```python
from build123d import *

# Parameters (mm, degrees)
EXTRUDE_1_DEPTH      = 3
SKETCH_2_R           = 1.5
CUT_EXTRUDE_1_DEPTH  = 3
SKETCH_3_R           = 18.5
SKETCH_3_R_2         = 1.5
CUT_EXTRUDE_2_DEPTH  = 10
SKETCH_4_W           = 90
SKETCH_4_H           = 90
CUT_EXTRUDE_3_DEPTH  = 3
FILLET_3_R           = 6
CHAMFER_1_SIZE       = 8
CUT_EXTRUDE_6_DEPTH  = 10
CHAMFER_2_SIZE       = 15
SKETCH_8_R           = 1.5
CUT_EXTRUDE_7_DEPTH  = 10
SKETCH_9_R           = 1.5
CUT_EXTRUDE_8_DEPTH  = 10
CUT_EXTRUDE_9_DEPTH  = 10
SKETCH_14_R          = 1.5
CUT_EXTRUDE_10_DEPTH = 10
SKETCH_15_R          = 1.5
SKETCH_15_W          = 42
SKETCH_15_H          = 23
CUT_EXTRUDE_11_DEPTH = 10
FILLET_4_R           = 1
SKETCH_16_R          = 1.25
CUT_EXTRUDE_12_DEPTH = 10
SKETCH_19_R          = 1.5
CUT_EXTRUDE_13_DEPTH = 10
SKETCH_20_R          = 1.5
CUT_EXTRUDE_14_DEPTH = 10
SKETCH_21_R          = 1.5
CUT_EXTRUDE_15_DEPTH = 10
SKETCH_22_R          = 1.5
CUT_EXTRUDE_16_DEPTH = 10


with BuildPart() as part:
    # 草图1 → 凸台-拉伸1 (new body)
    with BuildSketch(Plane(origin=(0, 0, 0), x_dir=(1, 0, 0), z_dir=(0, 1, 0))):
        Polygon((-47.5, -71), (-47.5, -125), (47.5, -125), (47.5, -71), (145, -71), (145, 71), (47.5, 71), (47.5, 125), (-47.5, 125), (-47.5, 71), (-145, 71), (-145, -71), align=None)
    extrude(amount=EXTRUDE_1_DEPTH)

    # 草图2 → 切除-拉伸1 (cut)
    with BuildSketch(Plane(origin=(0, 3, 0), x_dir=(1, 0, 0), z_dir=(0, 1, 0))):
        with Locations(Location((110, 62, 0), (0, 0, 270))):
            Circle(SKETCH_2_R)
        with Locations(Location((80, 62, 0), (0, 0, 270))):
            Circle(SKETCH_2_R)
        with Locations(Location((80, 38, 0), (0, 0, 270))):
            Circle(SKETCH_2_R)
        with Locations(Location((110, 38, 0), (0, 0, 270))):
            Circle(SKETCH_2_R)
        with Locations(Location((110, -38, 0), (0, 0, 90))):
            Circle(SKETCH_2_R)
        with Locations(Location((110, -62, 0), (0, 0, 90))):
            Circle(SKETCH_2_R)
        with Locations(Location((80, -38, 0), (0, 0, 90))):
            Circle(SKETCH_2_R)
        with Locations(Location((80, -62, 0), (0, 0, 90))):
            Circle(SKETCH_2_R)
        with Locations(Location((-80, -62, 0), (0, 0, 270))):
            Circle(SKETCH_2_R)
        with Locations(Location((-80, -38, 0), (0, 0, 270))):
            Circle(SKETCH_2_R)
        with Locations(Location((-110, -62, 0), (0, 0, 270))):
            Circle(SKETCH_2_R)
        with Locations(Location((-110, -38, 0), (0, 0, 270))):
            Circle(SKETCH_2_R)
        with Locations(Location((-110, 38, 0), (0, 0, 90))):
            Circle(SKETCH_2_R)
        with Locations(Location((-80, 38, 0), (0, 0, 90))):
            Circle(SKETCH_2_R)
        with Locations(Location((-80, 62, 0), (0, 0, 90))):
            Circle(SKETCH_2_R)
        with Locations(Location((-110, 62, 0), (0, 0, 90))):
            Circle(SKETCH_2_R)
    extrude(amount=-CUT_EXTRUDE_1_DEPTH, mode=Mode.SUBTRACT)

    # 草图3 → 切除-拉伸2 (cut)
    with BuildSketch(Plane(origin=(0, 3, 0), x_dir=(1, 0, 0), z_dir=(0, 1, 0))):
        with Locations(Location((0, 97, 0), (0, 0, 270))):
            Circle(SKETCH_3_R)
        with Locations(Location((29, 117, 0), (0, 0, 270))):
            Circle(SKETCH_3_R_2)
        with Locations(Location((29, 77, 0), (0, 0, 270))):
            Circle(SKETCH_3_R_2)
        with Locations(Location((-29, 77, 0), (0, 0, 270))):
            Circle(SKETCH_3_R_2)
        with Locations(Location((-29, 117, 0), (0, 0, 270))):
            Circle(SKETCH_3_R_2)
    extrude(amount=-CUT_EXTRUDE_2_DEPTH, mode=Mode.SUBTRACT)

    # 草图4 → 切除-拉伸3 (cut)
    with BuildSketch(Plane(origin=(0, 3, 0), x_dir=(1, 0, 0), z_dir=(0, 1, 0))):
        Rectangle(SKETCH_4_W, SKETCH_4_H)
    extrude(amount=-CUT_EXTRUDE_3_DEPTH, mode=Mode.SUBTRACT)

    # 圆角3
    fillet_3_edges = [part.edges().sort_by_distance(p)[0] for p in [
        (-145, 1.5, 71),
        (-145, 1.5, -71),
        (-47.5, 1.5, -125),
        (47.5, 1.5, -125),
        (145, 1.5, -71),
        (145, 1.5, 71),
        (47.5, 1.5, 125),
        (-47.5, 1.5, 125),
    ]]
    fillet(fillet_3_edges, radius=FILLET_3_R)

    # 倒角1
    chamfer_1_edges = [part.edges().sort_by_distance(p)[0] for p in [
        (-47.5, 1.5, 71),
        (-47.5, 1.5, -71),
        (47.5, 1.5, -71),
        (47.5, 1.5, 71),
    ]]
    chamfer(chamfer_1_edges, length=CHAMFER_1_SIZE)

    # 草图7 → 切除-拉伸6 (cut)
    with BuildSketch(Plane(origin=(0, 3, 0), x_dir=(1, 0, 0), z_dir=(0, 1, 0))):
        with BuildLine():
            Line((-65, -20), (-65, 20))
            ThreePointArc((-65, 20), (-58, 27), (-51, 20))
            Line((-51, 20), (-51, -20))
            ThreePointArc((-51, -20), (-58, -27), (-65, -20))
        make_face()
        with BuildLine():
            Line((-141, -15), (-141, 15))
            ThreePointArc((-141, 15), (-137, 19), (-133, 15))
            Line((-133, 15), (-133, -15))
            ThreePointArc((-133, -15), (-137, -19), (-141, -15))
        make_face()
        with BuildLine():
            Line((129, 38), (129, 52))
            ThreePointArc((129, 52), (134, 57), (139, 52))
            Line((139, 52), (139, 38))
            ThreePointArc((139, 38), (134, 33), (129, 38))
        make_face()
        with BuildLine():
            Line((129, -38), (129, -52))
            ThreePointArc((129, -52), (134, -57), (139, -52))
            Line((139, -52), (139, -38))
            ThreePointArc((139, -38), (134, -33), (129, -38))
        make_face()
    extrude(amount=-CUT_EXTRUDE_6_DEPTH, mode=Mode.SUBTRACT)

    # 倒角2
    chamfer_2_edges = [part.edges().sort_by_distance(p)[0] for p in [
        (45, 1.5, -45),
        (45, 1.5, 45),
        (-45, 1.5, 45),
        (-45, 1.5, -45),
    ]]
    chamfer(chamfer_2_edges, length=CHAMFER_2_SIZE)

    # 草图8 → 切除-拉伸7 (cut)
    with BuildSketch(Plane(origin=(0, 3, 0), x_dir=(1, 0, 0), z_dir=(0, 1, 0))):
        with Locations(Location((-139, 50, 0), (0, 0, 270))):
            Circle(SKETCH_8_R)
        with Locations(Location((-131, 50, 0), (0, 0, 270))):
            Circle(SKETCH_8_R)
    extrude(amount=-CUT_EXTRUDE_7_DEPTH, mode=Mode.SUBTRACT)

    # 草图9 → 切除-拉伸8 (cut)
    with BuildSketch(Plane(origin=(0, 3, 0), x_dir=(1, 0, 0), z_dir=(0, 1, 0))):
        with Locations(Location((50.843145751, 56.5, 0), (0, 0, 270))):
            Circle(SKETCH_9_R)
        with Locations(Location((56.5, 50.843145751, 0), (0, 0, 270))):
            Circle(SKETCH_9_R)
        with Locations(Location((56.5, -50.843145751, 0), (0, 0, 270))):
            Circle(SKETCH_9_R)
        with Locations(Location((50.843145751, -56.5, 0), (0, 0, 270))):
            Circle(SKETCH_9_R)
        with Locations(Location((-50.843145751, -56.5, 0), (0, 0, 270))):
            Circle(SKETCH_9_R)
        with Locations(Location((-56.5, -50.843145751, 0), (0, 0, 270))):
            Circle(SKETCH_9_R)
        with Locations(Location((-56.5, 50.843145751, 0), (0, 0, 270))):
            Circle(SKETCH_9_R)
        with Locations(Location((-50.843145751, 56.5, 0), (0, 0, 270))):
            Circle(SKETCH_9_R)
        with Locations(Location((-38, -117, 0), (0, 0, 270))):
            Circle(SKETCH_9_R)
        with Locations(Location((38, -117, 0), (0, 0, 270))):
            Circle(SKETCH_9_R)
    extrude(amount=-CUT_EXTRUDE_8_DEPTH, mode=Mode.SUBTRACT)

    # 草图12 → 切除-拉伸9 (cut)
    with BuildSketch(Plane(origin=(0, 3, 0), x_dir=(1, 0, 0), z_dir=(0, 1, 0))):
        with BuildLine():
            Line((-17.5, -54), (17.5, -54))
            ThreePointArc((17.5, -54), (23.5, -60), (17.5, -66))
            Line((17.5, -66), (-17.5, -66))
            ThreePointArc((-17.5, -66), (-23.5, -60), (-17.5, -54))
        make_face()
    extrude(amount=-CUT_EXTRUDE_9_DEPTH, mode=Mode.SUBTRACT)

    # 草图14 → 切除-拉伸10 (cut)
    with BuildSketch(Plane(origin=(0, 3, 0), x_dir=(1, 0, 0), z_dir=(0, 1, 0))):
        with Locations(Location((36, -69, 0), (0, 0, 270))):
            Circle(SKETCH_14_R)
        with Locations(Location((36, -111, 0), (0, 0, 270))):
            Circle(SKETCH_14_R)
        with Locations(Location((-36, -111, 0), (0, 0, 270))):
            Circle(SKETCH_14_R)
        with Locations(Location((-36, -69, 0), (0, 0, 270))):
            Circle(SKETCH_14_R)
    extrude(amount=-CUT_EXTRUDE_10_DEPTH, mode=Mode.SUBTRACT)

    # 草图15 → 切除-拉伸11 (cut)
    with BuildSketch(Plane(origin=(0, 3, 0), x_dir=(1, 0, 0), z_dir=(0, 1, 0))):
        with Locations(Location((75.36, 5, 0), (0, 0, 270))):
            Circle(SKETCH_15_R)
        with Locations(Location((75.36, -5, 0), (0, 0, 270))):
            Circle(SKETCH_15_R)
        with Locations(Location((124.86, -5, 0), (0, 0, 270))):
            Circle(SKETCH_15_R)
        with Locations(Location((124.86, 5, 0), (0, 0, 270))):
            Circle(SKETCH_15_R)
        with Locations((100.11, 0)):
            Rectangle(SKETCH_15_W, SKETCH_15_H)
    extrude(amount=-CUT_EXTRUDE_11_DEPTH, mode=Mode.SUBTRACT)

    # 圆角4
    fillet_4_edges = [part.edges().sort_by_distance(p)[0] for p in [
        (121.11, 1.5, -11.5),
        (121.11, 1.5, 11.5),
        (79.11, 1.5, 11.5),
        (79.11, 1.5, -11.5),
    ]]
    fillet(fillet_4_edges, radius=FILLET_4_R)

    # 草图16 → 切除-拉伸12 (cut)
    with BuildSketch(Plane(origin=(0, 3, 0), x_dir=(1, 0, 0), z_dir=(0, 1, 0))):
        with Locations(Location((-73.5, 37, 0), (0, 0, 270))):
            Circle(SKETCH_16_R)
        with Locations(Location((-122.5, 37, 0), (0, 0, 270))):
            Circle(SKETCH_16_R)
        with Locations(Location((-73.5, -21, 0), (0, 0, 270))):
            Circle(SKETCH_16_R)
        with Locations(Location((-122.5, -21, 0), (0, 0, 270))):
            Circle(SKETCH_16_R)
    extrude(amount=-CUT_EXTRUDE_12_DEPTH, mode=Mode.SUBTRACT)

    # 草图19 → 切除-拉伸13 (cut)
    with BuildSketch(Plane(origin=(0, 3, 0), x_dir=(1, 0, 0), z_dir=(0, 1, 0))):
        with Locations(Location((-65, 50, 0), (0, 0, 270))):
            Circle(SKETCH_19_R)
        with Locations(Location((-131, 50, 0), (0, 0, 270))):
            Circle(SKETCH_19_R)
        with Locations(Location((-65, -64.8, 0), (0, 0, 270))):
            Circle(SKETCH_19_R)
        with Locations(Location((-131, -64.8, 0), (0, 0, 270))):
            Circle(SKETCH_19_R)
    extrude(amount=-CUT_EXTRUDE_13_DEPTH, mode=Mode.SUBTRACT)

    # 草图20 → 切除-拉伸14 (cut)
    with BuildSketch(Plane(origin=(0, 3, 0), x_dir=(1, 0, 0), z_dir=(0, 1, 0))):
        with Locations(Location((-60, 60, 0), (0, 0, 270))):
            Circle(SKETCH_20_R)
    extrude(amount=-CUT_EXTRUDE_14_DEPTH, mode=Mode.SUBTRACT)

    # 草图21 → 切除-拉伸15 (cut)
    with BuildSketch(Plane(origin=(0, 3, 0), x_dir=(1, 0, 0), z_dir=(0, 1, 0))):
        with Locations(Location((31, -84, 0), (0, 0, 270))):
            Circle(SKETCH_21_R)
        with Locations(Location((32, -117.5, 0), (0, 0, 270))):
            Circle(SKETCH_21_R)
        with Locations(Location((-28, -87.5, 0), (0, 0, 270))):
            Circle(SKETCH_21_R)
        with Locations(Location((-28, -117.5, 0), (0, 0, 270))):
            Circle(SKETCH_21_R)
    extrude(amount=-CUT_EXTRUDE_15_DEPTH, mode=Mode.SUBTRACT)

    # 草图22 → 切除-拉伸16 (cut)
    with BuildSketch(Plane(origin=(0, 3, 0), x_dir=(1, 0, 0), z_dir=(0, 1, 0))):
        with Locations(Location((73, 13, 0), (0, 0, 270))):
            Circle(SKETCH_22_R)
        with Locations(Location((49, 13, 0), (0, 0, 270))):
            Circle(SKETCH_22_R)
        with Locations(Location((73, -13, 0), (0, 0, 270))):
            Circle(SKETCH_22_R)
        with Locations(Location((49, -13, 0), (0, 0, 270))):
            Circle(SKETCH_22_R)
    extrude(amount=-CUT_EXTRUDE_16_DEPTH, mode=Mode.SUBTRACT)


solid = part.part
```
Can you work these out from the model? Positions are in its coordinate system, mm. A direction names the side the tool comes from. Coordinates: 2 decimals unless noted, no trailing zeros. Loops run counter-clockwise (first coordinate to the right, second up) from the corner with the lowest first, then second, coordinate; pieces in that order, holes last.
Item 1: Suppose I cut it at B-B (z = 100.5). Please give me the cut outline in (x, y), then the cut area to 3 significant figures.
Answers below:
outline: (-47.5, 0) - (47.5, 0) - (47.5, 3) - (-47.5, 3) - close
area: 285 mm2
Item 2: Suppose I cut it at C-C (y = 0.8). State how many separate pieces and enclosed holes the cut face has, then the cut area to 3 significant figures.
Answers below:
separate pieces: 1
enclosed holes: 64
area: 39,500 mm2
Item 3: Which directions (+Z, -Z, +X, -X, +Y, -Y) give clear straight access to the entire face, cutting with the end or side of a thin tool? Please do faces 4 (the face through (51.4, 1.5, -75.1)), 5 (the face through (-37, 2, -38)).
Answers below:
face 4: -Z, +X, +Y, -Y
face 5: +Y, -Y
Item 4: If we mould it in two halves opening along X, with no side actions, what happens to faces 1 (the face through (-23.5, 1.5, 60.1)), 2 (the face through (-2, 0, 53.8)), 3 (the face through (143.196, 1.521, 69.289))? For each: released by +X, released by -X, zero draft, split by the parting line, or undercut.
Answers below:
face 1: undercut
face 2: zero draft
face 3: released by +X
Item 5: Suppose I cut it at A-A (x = -3.5). Please give me the cut outline in (y, z), then the cut area to 3 significant figures.
Answers below:
outline: (0, -125) - (3, -125) - (3, -115.17) - (0, -115.17) - close; (0, -78.83) - (3, -78.83) - (3, -45) - (0, -45) - close; (0, 45) - (3, 45) - (3, 54) - (0, 54) - close; (0, 66) - (3, 66) - (3, 125) - (0, 125) - close
area: 335 mm2
Item 6: Please list where these lines run through material, in increasing order: L1, parallel to X at y = 1.55, z = 13; L2, parallel to Z at x = -80, y = 1.6; L3, parallel to Z at x = 80, y = 0.65.
Answers below:
L1: x = -145 to -141, -133 to -65, -51 to -45, 45 to 47.5, 50.5 to 71.5, 74.5 to 145
L2: z = -71 to -63.5, -60.5 to -39.5, -36.5 to 36.5, 39.5 to 60.5, 63.5 to 71
L3: z = -71 to -63.5, -60.5 to -39.5, -36.5 to -11.49, 11.49 to 36.5, 39.5 to 60.5, 63.5 to 71
Item 7: Suppose I cut it at D-D (x = -117). Please give me the cut outline in (y, z).
Answers below:
outline: (0, -71) - (3, -71) - (3, 71) - (0, 71) - close
Item 8: I'm going to push flat-ended pins straight in: pin 1 (3.5 mm diameter, centred on x = -36, z = 111, fed in from -Y); pin 2 (2.5 mm diameter, centred on x = -80, z = 38, fed in from -Y); pin 3 (1.5 mm diameter, centred on x = 90.5, y = 1, fed in from -Z). Where does each tip first touch, or does it pass through?
Answers below:
pin 1: stops at y = 0
pin 2: passes through
pin 3: stops at z = -71
